Model file for the job. Use its own axes, mm. Give positions to 0.01 mm unless a question says otherwise; leave off trailing zeros. Loops run counter-clockwise (first coordinate to the right, second up) from the corner with the lowest first, then second, coordinate; pieces in that order, holes last. Notation, with made-up numbers: M 41,18.5 L 62,18.5 A23 ccw 62,49.5 Z; hole C 65,-12 d2. An arc over 180 degrees is marked long. Use CSV: the item, a comma, the result in double quotes. Start each with the question number.
(1) Slice it at B-B on x = 25. List the corners of the cut face in (y, z), and give its area (3 significant figures).
(2) Two-plate mould, pull along Y, no slides. Class faces 1 (the face through (0, -10, 5)), 2 (the face through (0, 90, 5)), 3 (the face through (-28.31, 1.04, 6.75)): pulls with the +Y half, pulls with the -Y half, needs draft (parallel to the pull), parting line crosses it, or undercut.
(3) Slice it at A-A on y = 0. List the corners of the cut face in (x, z).
(4) Flat gauge pin, fed straight in: P1, Ø6, axis at x = 25, y = 0, coming from the +Z side. Where does the tip first touch, or does it go through?
(5) Slice it at C-C on z = 8.25. List the corners of the cut face in (x, y).
(6) Wall check: line 1 along X through (y, z) = (0, 2.5); line 2 along Y through (x, z) = (25, 4); line 3 along X through (y, z) = (-1.5, 5). Give the ranges that are in metal, low to high. Write a range as from..to.
```python
from build123d import *

# Parameters (mm, degrees)
F0_W           = 70
F0_H           = 100
F1_DEPTH       = 10
F3_D           = 6.6
F3_CSINK_D     = 13.44
F3_CSINK_ANGLE = 90


# Not quite as in the source:
# - a pattern or mirror of a feature is missing from the dataset's text; its kind, count and spacing are read off the source's solid


with BuildPart() as f1:
    # F0 (on Top) → F1 (new body)
    with BuildSketch(Plane.XY):
        with Locations((0, 40)):
            Rectangle(F0_W, F0_H)
    extrude(amount=F1_DEPTH)

    # F3 (through all)
    with Locations(Plane.XY.offset(10)):
        with Locations((-25, 0)):
            f3 = CounterSinkHole(F3_D / 2, F3_CSINK_D / 2, counter_sink_angle=F3_CSINK_ANGLE)

    # F3_copies: F3 across plane
    add(f3.mirror(Plane(origin=(0, 0, 0), x_dir=(0, 0, 1), z_dir=(1, 0, 0))), mode=Mode.SUBTRACT)


solid = f1.part
```
Reply:
1,outline,"M -10,0 L -3.3,0 L -3.3,6.58 L -6.72,10 L -10,10 Z; M 3.3,0 L 90,0 L 90,10 L 6.72,10 L 3.3,6.58 Z"
1,area,"922 mm^2"
2,face 1,"pulls with the -Y half"
2,face 2,"pulls with the +Y half"
2,face 3,"undercut"
3,outline,"M -35,0 L -28.3,0 L -28.3,6.58 L -31.72,10 L -35,10 Z; M -21.7,0 L 21.7,0 L 21.7,6.58 L 18.28,10 L -18.28,10 L -21.7,6.58 Z; M 28.3,0 L 35,0 L 35,10 L 31.72,10 L 28.3,6.58 Z"
4,P1,"passes through"
5,outline,"M -35,-10 L 35,-10 L 35,90 L -35,90 Z; hole C -25,0 d9.94; hole C 25,0 d9.94"
6,line 1,"x = -35..-28.3, -21.7..21.7, 28.3..35"
6,line 2,"y = -10..-3.3, 3.3..90"
6,line 3,"x = -35..-27.94, -22.06..22.06, 27.94..35"
